Read the model definition and answer for the solid it produces. Units are mm, in the model's axes. A direction names the side the tool comes from. Coordinates: 2 decimals unless noted, no trailing zeros. Loops run counter-clockwise (first coordinate to the right, second up) from the corner with the lowest first, then second, coordinate; pieces in that order, holes last.
from build123d import *

# Parameters (mm, degrees)
F0_R          = 23.1775
F1_DEPTH      = 46.7106
F2_R          = 10.4599637804
F3_DEPTH      = 63.5
F5_DEPTH      = 23.1785
F5_DEPTH_BACK = 23.1785


with BuildPart() as f1:
    # F0 (on Top) → F1 (new body)
    with BuildSketch(Plane.XY):
        Circle(F0_R)
    extrude(amount=F1_DEPTH)

    # F2 (on face) → F3 (join)
    with BuildSketch(Plane.XY.offset(46.7106)):
        Circle(F2_R)
    extrude(amount=F3_DEPTH)

    # F4 (on Front) → F5 (cut, two sides)
    with BuildSketch(Plane.XZ) as f5_sk:
        Polygon((-10.4648, 5.8166), (-16.2814, 0), (23.1775, 0), (23.1775, 5.8166), align=None)
    extrude(amount=-F5_DEPTH, mode=Mode.SUBTRACT)
    extrude(f5_sk.sketch, amount=F5_DEPTH_BACK, mode=Mode.SUBTRACT)


solid = f1.part
Q1. Determine the mould class of faces 3 (the face through (3, 0, 5.817)), 4 (the face through (-13.33, -0.29, 2.95)), 5 (the face through (-23.155, 1.019, 23.028)) for opening direction X: +X half, -X half, draft (parallel to the pull), parting line (faces both ways), or undercut.
Findings below:
face 3: draft
face 4: +X half
face 5: parting line
Q2. Flat-ended cylindrical pins translate along their axes: pin 1 Ø10 at (x, y) = (-3.5, 3.5) entering from -Z; pin 2 Ø3 at (y, z) = (-9.5, 55) entering from +X; pin 3 Ø2 at (x, z) = (-3.5, 56) entering from -Y. Find the tip coordinate at first contact, or state that the pin passes through.
Findings below:
pin 1: stops at z = 5.82
pin 2: stops at x = 6.74
pin 3: stops at y = -10.16
Q3. A cutting plane is placed at C-C (z = 62). Give the vertices of the cut face in (x, y).
Findings below:
outline: circle Ø20.92 at (0, 0)
Q4. Which of the six approach directions +Z, -Z, +X, -X, +Y, -Y give full straight-line access (tool end or side, diameter ignored) to faces 1 (the face through (-19, 0, 0)), 2 (the face through (9.977, 3.142, 78.016))?
Findings below:
face 1: -Z, +X, -X, +Y, -Y
face 2: +Z
Q5. A cutting plane is placed at D-D (y = 9). Give the vertices of the cut face in (x, z).
Findings below:
outline: (-21.36, 0) - (-16.28, 0) - (-10.46, 5.82) - (21.36, 5.82) - (21.36, 46.71) - (5.33, 46.71) - (5.33, 110.21) - (-5.33, 110.21) - (-5.33, 46.71) - (-21.36, 46.71) - close
Q6. Straight lines are drawn through the part: probe 1 along Z at (x, y) = (-20, 11); probe 2 along Z at (x, y) = (15, -6.5); probe 3 along Y at (x, z) = (10.5, 11). For each, find the intervals that lie inside material, in ascending order.
Findings below:
probe 1: z = 0 to 46.71
probe 2: z = 5.82 to 46.71
probe 3: y = -20.66 to 20.66
Q7. A cutting plane is placed at A-A (x = 0). Give the vertices of the cut face in (y, z).
Findings below:
outline: (-23.18, 5.82) - (23.18, 5.82) - (23.18, 46.71) - (10.46, 46.71) - (10.46, 110.21) - (-10.46, 110.21) - (-10.46, 46.71) - (-23.18, 46.71) - close
Q8. A cutting plane is placed at B-B (y = 0). Give the vertices of the cut face in (x, z).
Findings below:
outline: (-23.18, 0) - (-16.28, 0) - (-10.46, 5.82) - (23.18, 5.82) - (23.18, 46.71) - (10.46, 46.71) - (10.46, 110.21) - (-10.46, 110.21) - (-10.46, 46.71) - (-23.18, 46.71) - close
